Can you work these out from the model? Positions are in its coordinate system, mm. Face numbers are marked on the shaded views. A direction names the side the tool comes from. Give positions to 0.01 mm unless a question says otherwise; leave off trailing zeros. Order: outer loops, then holes, each group sorted by start corner. A loop starts at its lowest first (then second) coordinate and runs counter-clockwise, first axis right, second up. Notation, with made-up numbers: M -10.5,38 L 13.5,38 A27 ccw 13.5,68 Z; hole C -3.75,-12 d5. An arc over 180 degrees is marked long. Use one line per item in the form item = value. Start each with the question number.
1. For the marked faces 5 and 6, which set-ups out of +Z, -Z, +X, -X, +Y, -Y let a thin tool reach every point of the face, with its end or its side?
2. I want a section at C-C, the plane x = 45.5. List the corners of the cut face in (y, z) for me (3 decimals).
3. We'd pull the mould along Z, two halves only. Please class the marked faces 1, 2, 3 and 4: +Z half, -Z half, draft (parallel to the pull), parting line (faces both ways), or undercut.
4. I want a section at A-A, the plane y = 47.5. Count the separate pieces of the cut face and the enclosed holes in it, and give its area (3 significant figures).
5. Will these pins go through, and if not, where does the flat tip stop? P1, Ø3, axis at x = 22.5, z = 28, coming from the +Y side; P2, Ø8, axis at x = 32, z = 33, coming from the +Y side; P3, Ø4, axis at x = 7.94, z = 38.1, coming from the +Y side; P4, Ø3, axis at x = 7.5, z = 12.5, coming from the +Y side.
6. I need wall thicknesses on L1, parallel to X at y = 45.75, z = 25.4 (3 decimals); L2, parallel to X at y = 41, z = 46 (3 decimals); L3, parallel to X at y = 45, z = 35.5 (3 decimals). Which ranges of each line are inside material? Lowest first, please.
7. I want a section at B-B, the plane y = 23. List the corners of the cut face in (x, z) for me (3 decimals), and give its area (3 significant figures).
```python
from build123d import *

# Parameters (mm, degrees)
EXTRUDE1_DEPTH                    = 50.8
SKETCH3_R                         = 1.5875
CUT_EXTRUDE2_DEPTH                = 7.62
CHAMFER3_SIZE                     = 0.762
CHAMFER3_SIZE2                    = 1.268180966
CHAMFER4_SIZE                     = 0.762
SKETCH4_R                         = 6.3627
CUT_EXTRUDE3_DEPTH                = 51.8
F_1_4_20_TAPPED_HOLE1_D           = 5.1054
F_1_4_20_TAPPED_HOLE1_DEPTH       = 16.51
F_1_4_20_TAPPED_HOLE1_CBORE_D     = 6.35
F_1_4_20_TAPPED_HOLE1_CBORE_DEPTH = 12.7
F_1_4_20_TAPPED_HOLE1_TIP         = 1.533816902
CHAMFER6_SIZE                     = 0.762
CHAMFER6_SIZE2                    = 1.319822715
CHAMFER7_SIZE                     = 0.762
CHAMFER7_SIZE2                    = 0.662396494
CHAMFER7_PART_2_SIZE              = 0.762
CHAMFER7_PART_2_SIZE2             = 0.662396494


with BuildPart() as part:
    # Sketch1 → Extrude1 (new body)
    with BuildSketch(Plane.XY):
        Polygon((0, 0), (50.8, 0), (50.8, 50.8), (34.9504, 50.8), (34.9504, 19.05), (15.875, 19.05), (15.875, 50.8), (0, 50.8), align=None)
    extrude(amount=EXTRUDE1_DEPTH)

    # Sketch3 → Cut-Extrude2 (cut)
    with BuildSketch(Plane(origin=(0, 50.8, 0), x_dir=(-1, 0, 0), z_dir=(0, 1, 0))):
        with Locations(Location((-7.9375, 25.4, 0), (0, 0, 90))):  # turned: the seam where the file's is
            Circle(SKETCH3_R)
    extrude(amount=-CUT_EXTRUDE2_DEPTH, mode=Mode.SUBTRACT)

    # Chamfer3
    chamfer3_edges = [part.edges().sort_by_distance(p)[0] for p in [
        (7.9375, 43.18, 23.8125),
    ]]
    chamfer3_side = [part.faces().sort_by_distance(p)[0] for p in [
        (7.9375, 46.99, 23.8125),
    ]]
    chamfer(chamfer3_edges, length=CHAMFER3_SIZE, length2=CHAMFER3_SIZE2, reference=chamfer3_side[0])

    # Chamfer4
    chamfer4_edges = [part.edges().sort_by_distance(p)[0] for p in [
        (7.9375, 50.8, 23.8125),
    ]]
    chamfer(chamfer4_edges, length=CHAMFER4_SIZE)

    # Sketch4 → Cut-Extrude3 (cut, through all)
    with BuildSketch(Plane(origin=(50.8, 0, 0), x_dir=(0, 0, -1), z_dir=(1, 0, 0))):
        with Locations(Location((-25.4, 34.925, 0), (0, 0, 90))):  # turned: the seam where the file's is
            Circle(SKETCH4_R)
    extrude(amount=-CUT_EXTRUDE3_DEPTH, mode=Mode.SUBTRACT)

    # 1/4-20 Tapped Hole1
    with Locations(Plane(origin=(7.9375, 50.8, 12.7), x_dir=(0, 0, 1), z_dir=(0, 1, 0))):
        with Locations((0, 0), (25.4, 0)):
            CounterBoreHole(F_1_4_20_TAPPED_HOLE1_D / 2, F_1_4_20_TAPPED_HOLE1_CBORE_D / 2, F_1_4_20_TAPPED_HOLE1_CBORE_DEPTH, depth=F_1_4_20_TAPPED_HOLE1_DEPTH)
            with Locations((0, 0, -(F_1_4_20_TAPPED_HOLE1_DEPTH + F_1_4_20_TAPPED_HOLE1_TIP / 2))):  # 118° drill point
                Cone(0, F_1_4_20_TAPPED_HOLE1_D / 2, F_1_4_20_TAPPED_HOLE1_TIP, mode=Mode.SUBTRACT)

    # Chamfer6
    chamfer6_edges = [part.edges().sort_by_distance(p)[0] for p in [
        (7.9375, 50.8, 34.925),
        (7.9375, 50.8, 9.525),
    ]]
    chamfer6_side = [part.faces().sort_by_distance(p)[0] for p in [
        (15.342773016, 50.8, 25.4),
    ]]
    chamfer(chamfer6_edges, length=CHAMFER6_SIZE, length2=CHAMFER6_SIZE2, reference=chamfer6_side[0])

    # Chamfer7
    chamfer7_edges = [part.edges().sort_by_distance(p)[0] for p in [
        (0, 28.5623, 25.4),
    ]]
    chamfer7_side = [part.faces().sort_by_distance(p)[0] for p in [
        (7.9375, 28.5623, 25.4),
    ]]
    chamfer(chamfer7_edges, length=CHAMFER7_SIZE, length2=CHAMFER7_SIZE2, reference=chamfer7_side[0])

    # Chamfer7 part 2
    chamfer7_part_2_edges = [part.edges().sort_by_distance(p)[0] for p in [
        (50.8, 28.5623, 25.4),
    ]]
    chamfer7_part_2_side = [part.faces().sort_by_distance(p)[0] for p in [
        (50.8, 24.906235921, 25.4),
    ]]
    chamfer(chamfer7_part_2_edges, length=CHAMFER7_PART_2_SIZE, length2=CHAMFER7_PART_2_SIZE2, reference=chamfer7_part_2_side[0])


solid = part.part
```
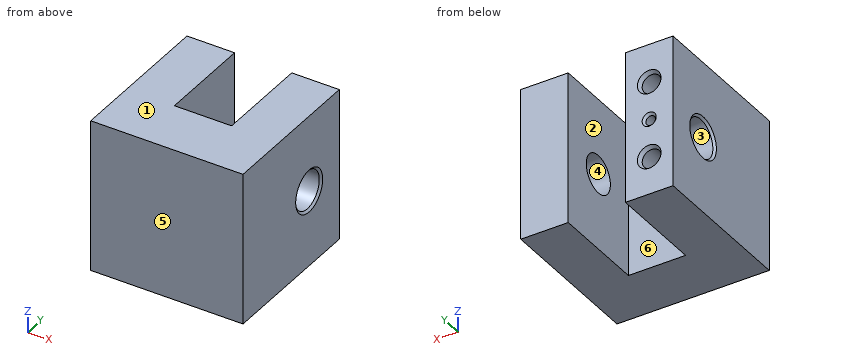
Check result:
q1.face_5 = +Z, -Z, +X, -X, -Y
q1.face_6 = +Z, -Z, +Y
q2.outline = M 0,0 L 50.8,0 L 50.8,50.8 L 0,50.8 Z; hole C 34.925,25.4 d12.725
q3.face_1 = +Z half
q3.face_2 = draft
q3.face_3 = undercut
q3.face_4 = undercut
q4.separate_pieces = 2
q4.enclosed_holes = 3
q4.area = 1,540 mm2
q5.P1 = 19.05
q5.P2 = 50.8
q5.P3 = 33.96
q5.P4 = 33.95
q6.L1 = 0 to 6.35, 9.525 to 15.875, 34.95 to 50.8
q6.L2 = 0 to 15.875, 34.95 to 50.8
q6.L3 = 0 to 6.115, 9.76 to 15.875, 34.95 to 50.8
q7.outline = M 0,0 L 15.875,0 L 15.875,50.8 L 0,50.8 Z; M 34.95,0 L 50.8,0 L 50.8,50.8 L 34.95,50.8 Z
q7.area = 1,610 mm2
